Here's how the part is built. I have some questions about the finished solid (model axes, mm). A direction names the side the tool comes from. Round coordinates to 2 decimals unless told otherwise and drop trailing zeros. Loops run counter-clockwise (first coordinate to the right, second up) from the corner with the lowest first, then second, coordinate; pieces in that order, holes last. Notation, with made-up numbers: (-31, 5.25) -> (-26, 5.25) arc R32 cw to (-26, 31.25) -> close; hole circle Ø10 at (11.25, -40). An arc over 180 degrees is marked (long way). One line per item, written item: value. Start each with the question number.
```python
from build123d import *

# Parameters (mm, degrees)
SKETCH2_W           = 57.15
SKETCH2_H           = 49.784
BOSS_EXTRUDE1_DEPTH = 14.224
SKETCH3_W           = 44.196
SKETCH3_H           = 39.37
CUT_EXTRUDE1_DEPTH  = 8.255
SKETCH4_W           = 35.56
SKETCH4_H           = 4.191
SKETCH4_W_2         = 15.621
SKETCH4_H_2         = 6.858
CUT_EXTRUDE2_DEPTH  = 8.255
SKETCH5_W           = 7.62
SKETCH5_H           = 8.89
SKETCH5_H_2         = 7.62
BOSS_EXTRUDE2_DEPTH = 6.604
SKETCH6_W           = 2.54
SKETCH6_H           = 5.08
SKETCH6_W_2         = 5.08
SKETCH6_H_2         = 2.54
CUT_EXTRUDE3_DEPTH  = 6.604
FILLET1_R           = 5.08
FILLET2_R           = 2.54
SKETCH7_W           = 127
SKETCH7_H           = 14.224
SKETCH7_R           = 2.38125
BOSS_EXTRUDE3_DEPTH = 5.207
BOSS_EXTRUDE4_DEPTH = 127
SKETCH11_W          = 34.925
SKETCH11_H          = 11.176
BOSS_EXTRUDE5_DEPTH = 5.207
SKETCH9_R           = 2.413
CUT_EXTRUDE4_DEPTH  = 25.4
FILLET3_R           = 5.08
FILLET4_R           = 5.08
BOSS_EXTRUDE6_DEPTH = 6.35
BOSS_EXTRUDE7_DEPTH = 6.35
BOSS_EXTRUDE8_DEPTH = 127
BOSS_EXTRUDE9_DEPTH = 127
CUT_EXTRUDE6_START  = -1.945752886
SKETCH16_R          = 2.413
CUT_EXTRUDE6_DEPTH  = 1.945752886
CUT_EXTRUDE9_START  = -22.261352
SKETCH17_R          = 5.08
CUT_EXTRUDE9_DEPTH  = 12.101352
FILLET5_R           = 3.81


with BuildPart() as part:
    # Sketch2 → Boss-Extrude1 (new body)
    with BuildSketch(Plane(origin=(0, 0, 0), x_dir=(1, 0, 0), z_dir=(0, 1, 0))):
        with Locations((28.575, 24.892)):
            Rectangle(SKETCH2_W, SKETCH2_H)
    extrude(amount=BOSS_EXTRUDE1_DEPTH)

    # Sketch3 → Cut-Extrude1 (cut)
    with BuildSketch(Plane(origin=(0, 14.224, 0), x_dir=(1, 0, 0), z_dir=(0, 1, 0))):
        with Locations((28.575, 24.892)):
            Rectangle(SKETCH3_W, SKETCH3_H)
    extrude(amount=-CUT_EXTRUDE1_DEPTH, mode=Mode.SUBTRACT)

    # Sketch4 → Cut-Extrude2 (cut)
    with BuildSketch(Plane(origin=(0, 5.969, 0), x_dir=(1, 0, 0), z_dir=(0, 1, 0))):
        with Locations((28.575, 12.5095)):
            Rectangle(SKETCH4_W, SKETCH4_H)
        with Locations((28.575, 24.638)):
            Rectangle(SKETCH4_W_2, SKETCH4_H_2)
    extrude(amount=-CUT_EXTRUDE2_DEPTH, mode=Mode.SUBTRACT)

    # Sketch5 → Boss-Extrude2 (add)
    with BuildSketch(Plane(origin=(0, 14.224, 0), x_dir=(1, 0, 0), z_dir=(0, 1, 0))):
        with Locations((-3.81, 24.765)):
            Rectangle(SKETCH5_W, SKETCH5_H)
        Polygon((12.7, 49.784), (36.83, 49.784), (44.45, 49.784), (44.45, 57.404), (36.83, 57.404), (12.7, 57.404), align=None)
        with Locations((60.96, 24.765)):
            Rectangle(SKETCH5_W, SKETCH5_H_2)
    extrude(amount=-BOSS_EXTRUDE2_DEPTH)

    # Sketch6 → Cut-Extrude3 (cut)
    with BuildSketch(Plane(origin=(0, 14.224, 0), x_dir=(1, 0, 0), z_dir=(0, 1, 0))):
        with Locations((-3.81, 24.765)):
            Rectangle(SKETCH6_W, SKETCH6_H)
        with Locations((60.96, 24.765)):
            Rectangle(SKETCH6_W, SKETCH6_H)
        with Locations((16.51, 53.594)):
            Rectangle(SKETCH6_W_2, SKETCH6_H_2)
        with Locations((40.64, 53.594)):
            Rectangle(SKETCH6_W_2, SKETCH6_H_2)
    extrude(amount=-CUT_EXTRUDE3_DEPTH, mode=Mode.SUBTRACT)

    # Fillet1
    fillet1_edges = [part.edges().sort_by_distance(p)[0] for p in [
        (0, 7.112, -49.784),
        (57.15, 7.112, -49.784),
        (57.15, 7.112, 0),
        (0, 7.112, 0),
    ]]
    fillet(fillet1_edges, radius=FILLET1_R)

    # Fillet2
    fillet2_edges = [part.edges().sort_by_distance(p)[0] for p in [
        (-7.62, 10.922, -20.32),
        (-7.62, 10.922, -29.21),
        (12.7, 10.922, -57.404),
        (44.45, 10.922, -57.404),
        (64.77, 10.922, -28.575),
        (64.77, 10.922, -20.955),
    ]]
    fillet(fillet2_edges, radius=FILLET2_R)

    # Sketch7 → Boss-Extrude3 (add)
    with BuildSketch(Plane.XY):
        with Locations((28.575, 7.112)):
            Rectangle(SKETCH7_W, SKETCH7_H)
        with Locations((-30.861, 7.112)):
            Circle(SKETCH7_R, mode=Mode.SUBTRACT)
        with Locations((88.011, 7.112)):
            Circle(SKETCH7_R, mode=Mode.SUBTRACT)
    extrude(amount=-BOSS_EXTRUDE3_DEPTH)

    # Sketch8 → Boss-Extrude4 (add)
    with BuildSketch(Plane.ZY.offset(34.925)):
        Polygon((0, 25.4), (21.313130632, 25.4), (0, 0), (-5.207, 0), (-5.207, 14.224), (0, 14.224), align=None)
    extrude(amount=-BOSS_EXTRUDE4_DEPTH)

    # Sketch11 → Boss-Extrude5 (add)
    with BuildSketch(Plane(origin=(0, 0, 0), x_dir=(-1, 0, 0), z_dir=(0, 0, -1))):
        with Locations((17.4625, 19.812)):
            Rectangle(SKETCH11_W, SKETCH11_H)
        with Locations((-74.6125, 19.812)):
            Rectangle(SKETCH11_W, SKETCH11_H)
    extrude(amount=BOSS_EXTRUDE5_DEPTH)

    # Sketch9 → Cut-Extrude4 (cut, symmetric)
    with BuildSketch(Plane(origin=(0, 0, 0), x_dir=(1, 0, 0), z_dir=(0, -0.6427876096865434, 0.7660444431189748))):
        with Locations(Location((-22.225, 15.377345149, 0), (0, 0, 270))):
            Circle(SKETCH9_R)
        with Locations(Location((79.375, 15.377345149, 0), (0, 0, 270))):
            Circle(SKETCH9_R)
    extrude(amount=CUT_EXTRUDE4_DEPTH, both=True, mode=Mode.SUBTRACT)

    # Fillet3
    fillet3_edges = [part.edges().sort_by_distance(p)[0] for p in [
        (44.45, 10.922, -49.784),
        (12.7, 10.922, -49.784),
    ]]
    fillet(fillet3_edges, radius=FILLET3_R - 0.0001)  # a hair under: the kernel refuses the full size

    # Fillet4
    fillet4_edges = [part.edges().sort_by_distance(p)[0] for p in [
        (57.15, 10.922, -20.955),
        (57.15, 10.922, -28.575),
        (0, 10.922, -29.21),
        (0, 10.922, -20.32),
    ]]
    fillet(fillet4_edges, radius=FILLET4_R - 0.0001)  # a hair under: the kernel refuses the full size

    # Sketch12 → Boss-Extrude6 (add)
    with BuildSketch(Plane.ZY):
        Polygon((-5.207, 25.4), (-15.24, 0), (-5.207, 0), align=None)
    extrude(amount=BOSS_EXTRUDE6_DEPTH)

    # Sketch13 → Boss-Extrude7 (add)
    with BuildSketch(Plane(origin=(57.15, 0, 0), x_dir=(0, 0, -1), z_dir=(1, 0, 0))):
        Polygon((5.207, 25.4), (15.875, 0), (5.207, 0), align=None)
    extrude(amount=BOSS_EXTRUDE7_DEPTH)

    # Sketch14 → Boss-Extrude8 (add)
    with BuildSketch(Plane.ZY.offset(34.925)):
        Polygon((-5.207, 0), (-5.207, -6.205460957), (0, 0), align=None)
    extrude(amount=-BOSS_EXTRUDE8_DEPTH)

    # Sketch15 → Boss-Extrude9 (add)
    with BuildSketch(Plane(origin=(92.075, 0, 0), x_dir=(0, 0, -1), z_dir=(1, 0, 0))):
        Polygon((5.207, -6.205460957), (2.667, -6.205460957), (-23.853130632, 25.4), (-21.313130632, 25.4), align=None)
    extrude(amount=-BOSS_EXTRUDE9_DEPTH)

    # Sketch16 → Cut-Extrude6 (cut)
    with BuildSketch(Plane(origin=(0, 0, 0), x_dir=(-1, 0, 0), z_dir=(0, 0.6427876096865434, -0.7660444431189748)).offset(CUT_EXTRUDE6_START)):
        with Locations(Location((-79.375, 15.377345149, 0), (0, 0, 270))):
            Circle(SKETCH16_R)
        with Locations(Location((22.225, 15.377345149, 0), (0, 0, 270))):
            Circle(SKETCH16_R)
    extrude(amount=CUT_EXTRUDE6_DEPTH, mode=Mode.SUBTRACT)

    # Sketch17 → Cut-Extrude9 (cut)
    with BuildSketch(Plane(origin=(0, -1.250705846, 1.490533186), x_dir=(1, 0, 0), z_dir=(0, -0.6427876096865434, 0.7660444431189747)).offset(CUT_EXTRUDE9_START)):
        with Locations(Location((79.375, 15.377345149, 0), (0, 0, 171.701605742))):
            Circle(SKETCH17_R)
        with Locations(Location((-22.225, 15.377345149, 0), (0, 0, 8.298394258))):
            Circle(SKETCH17_R)
    extrude(amount=CUT_EXTRUDE9_DEPTH, mode=Mode.SUBTRACT)

    # Fillet5
    fillet5_edges = [part.edges().sort_by_distance(p)[0] for p in [
        (-34.925, 25.4, 9.323065316),
        (92.075, 25.4, 9.323065316),
        (92.075, 9.597269522, -5.207),
        (-34.925, 9.597269522, -5.207),
    ]]
    fillet(fillet5_edges, radius=FILLET5_R)


solid = part.part
```
Q1. I want a section at D-D on z = -46.5. Please give me the cut outline in (x, y), plus the area to 3 significant figures.
Q2. If I drill on line 1 along X through (y, z) = (3.5, -11) (3 decimals); line 2 along X through (y, z) = (21, 6) (3 decimals); line 3 along Z through (x, y) = (8, 19.5), over which ranges is the centre line in solid material (lowest first)?
Q3. Will these pins go through, and if not, where does the flat tip stop? P1, Ø4.5, axis at y = 4.5, z = -11.5, coming from the +X side; P2, Ø0.8, axis at x = 61.5, y = 9.5, coming from the -Z side; P3, Ø1.5, axis at x = -5.5, z = -29, coming from the +Y side.
Q4. Which directions (+Z, -Z, +X, -X, +Y, -Y) give clear straight access to the entire face, cutting with the end or side of a thin tool? Please do faces 1 (the flat face through (63.5, 7, -8)), 2 (the flat face through (59, 7.62, -25)), 3 (the flat face through (57.15, 20, -4)), 4 (the flat face through (-4, 11, -22.225)), 5 (the flat face through (28, 10, -44.577)).
Q5. I want a section at C-C on z = -18.5. Please give me the cut outline in (x, y), plus the area to 3 significant figures.
Q6. I want a section at B-B on x = 9.5. Please give me the cut outline in (y, z).
Q7. If we mould it in two halves opening along Y, with no side actions, what happens to faces 6 (the flat face through (29, 25.4, 13)), 7 (the flat face through (36.386, 3, -25)), 8 (the cylindrical face through (-17.3, 19.2, -0.9))? For each: released by +Y, released by -Y, zero draft, split by the parting line, or undercut.
Q8. I want a section at A-A on y = 2.5. State how many separate pieces and enclosed holes the cut face has, plus the area to 3 significant figures.
Answers below:
1. outline: (0.33, 0) -> (56.82, 0) -> (56.82, 14.22) -> (0.33, 14.22) -> close
1. area: 804 mm^2
2. line 1: x = -6.35 to 10.795, 46.355 to 63.5
2. line 2: x = -34.925 to -24.451, -19.999 to 77.149, 81.601 to 92.075
2. line 3: z = 0 to 18.9
3. P1: stops at x = 63.5
3. P2: stops at z = -28.7
3. P3: stops at y = 14.22
4. face 1: +X, +Y, -Y
4. face 2: -Z, +X, -Y
4. face 3: -Z, +Y
4. face 4: +Y, -Y
4. face 5: +Y
5. outline: (-1.18, 7.62) -> (0, 7.62) -> (0, 0) -> (57.15, 0) -> (57.15, 7.62) -> (57.88, 7.62) -> (57.88, 14.22) -> (50.67, 14.22) -> (50.67, 5.97) -> (6.48, 5.97) -> (6.48, 14.22) -> (-1.18, 14.22) -> close
5. area: 461 mm^2
6. outline: (-6.21, -5.21) -> (0, -5.21) -> (0, -49.78) -> (7.62, -49.78) -> (7.62, -50.14) -> (14.22, -50.14) -> (14.22, -44.58) -> (5.97, -44.58) -> (5.97, -5.21) -> (14.22, -5.21) -> (14.22, 0) -> (25.4, 0) -> (25.4, 23.85) -> (-6.21, -2.67) -> close
7. face 6: released by +Y
7. face 7: zero draft
7. face 8: undercut
8. separate pieces: 1
8. enclosed holes: 2
8. area: 3,640 mm^2
